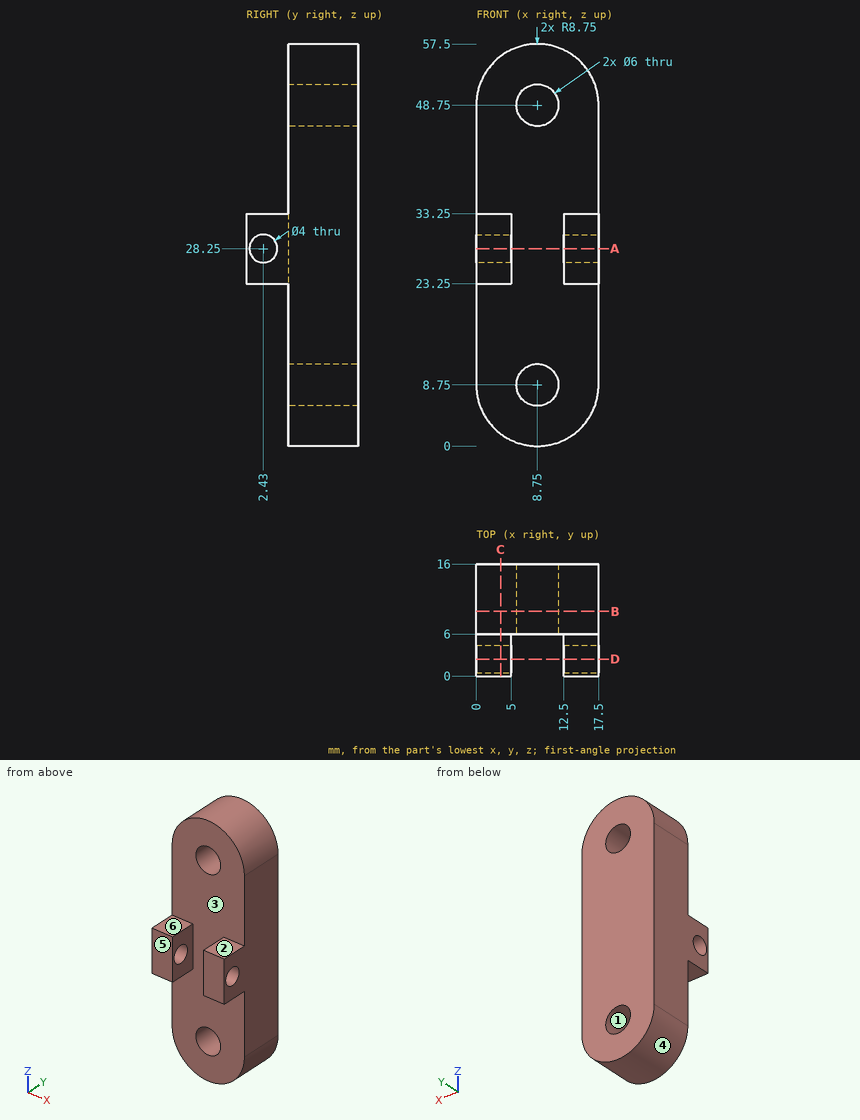
Print and shaded views of the part. All mm, measured from the part's lowest x, y and z. A direction names the side the tool comes from. Give positions to 0.01 mm unless a question says otherwise; leave off trailing zeros. Loops run counter-clockwise (first coordinate to the right, second up) from the corner with the lowest first, then second, coordinate; pieces in that order, holes last. Notation, with made-up numbers: (-9.5, -35) -> (45.5, -35) arc R10 ccw to (45.5, -20) -> close; hole circle Ø6 at (-23, 6.25). An arc over 180 degrees is marked (long way). Answer in a Markdown table with one row per item.
Item 1: Probe line 1 along Y through (x, z) = (2.1, 28.25); line 2 along X through (y, z) = (14.25, 8.75); line 3 along Z through (x, y) = (10.25, 12). List the from-to ranges inside material, lowest first. Write a range as [from, to].
Findings below:
| item | result |
|---|---|
| line 1 | y = [0, 0.43], [4.43, 16] |
| line 2 | x = [0, 5.75], [11.75, 17.5] |
| line 3 | z = [0.13, 6.15], [11.35, 46.15], [51.35, 57.37] |
Item 2: Slice it at D-D on y = 2.43. Write the cut outline in (x, z), plus the area to 3 significant figures.
Findings below:
| item | result |
|---|---|
| outline | (0, 23.25) -> (5, 23.25) -> (5, 26.25) -> (0, 26.25) -> close; (0, 30.25) -> (5, 30.25) -> (5, 33.25) -> (0, 33.25) -> close; (12.5, 23.25) -> (17.5, 23.25) -> (17.5, 26.25) -> (12.5, 26.25) -> close; (12.5, 30.25) -> (17.5, 30.25) -> (17.5, 33.25) -> (12.5, 33.25) -> close |
| area | 60.0 mm² |
Item 3: Flat gauge pins, fed straight in: P1, Ø6.5, axis at y = 2.43, z = 28.25, coming from the +X side; P2, Ø3, axis at x = 2.5, y = 5, coming from the -Z side; P3, Ø5.5, axis at x = 16, y = 2.5, coming from the +Z side; P4, Ø9.5, axis at x = 8.75, z = 48.75, coming from the -Y side. Where does each tip first touch, or does it go through?
Findings below:
| item | result |
|---|---|
| P1 | stops at x = 17.5 |
| P2 | stops at z = 1.66 |
| P3 | stops at z = 33.25 |
| P4 | stops at y = 6 |
Item 4: Mould opens along Z. For the marked faces 1, 2, 3 and 4 say: pulls with the +Z half, pulls with the -Z half, needs draft (parallel to the pull), parting line crosses it, or undercut.
Findings below:
| item | result |
|---|---|
| face 1 | undercut |
| face 2 | pulls with the +Z half |
| face 3 | needs draft |
| face 4 | pulls with the -Z half |
Item 5: Slice it at A-A on z = 28.25. Write the cut outline in (x, y).
Findings below:
| item | result |
|---|---|
| outline | (0, 0) -> (5, 0) -> (5, 0.43) -> (0, 0.43) -> close; (0, 4.43) -> (5, 4.43) -> (5, 6) -> (12.5, 6) -> (12.5, 4.43) -> (17.5, 4.43) -> (17.5, 16) -> (0, 16) -> close; (12.5, 0) -> (17.5, 0) -> (17.5, 0.43) -> (12.5, 0.43) -> close |
Item 6: Slice it at B-B on y = 9.25. Write the cut outline in (x, z).
Findings below:
| item | result |
|---|---|
| outline | (0, 8.75) arc R8.75 ccw to (17.5, 8.75) -> (17.5, 48.75) arc R8.75 ccw to (0, 48.75) -> close; hole circle Ø6 at (8.75, 8.75); hole circle Ø6 at (8.75, 48.75) |
Item 7: Slice it at C-C on x = 3.5. Write the cut outline in (y, z).
Findings below:
| item | result |
|---|---|
| outline | (0, 23.25) -> (6, 23.25) -> (6, 1.75) -> (16, 1.75) -> (16, 55.75) -> (6, 55.75) -> (6, 33.25) -> (0, 33.25) -> close; hole circle Ø4 at (2.43, 28.25) |
Item 8: Tool access for the marked faces 5 and 6: list every direction of +Z, -Z, +X, -X, +Y, -Y with a clear straight run to the whole face (end or side of a thin tool).
Findings below:
| item | result |
|---|---|
| face 5 | +Z, -Z, +X, -X, -Y |
| face 6 | +Z, +X, -X, -Y |
